Study the drawing (mm; zero at the part's minimum x, y, z) and answer. A direction names the side the tool comes from. Give positions to 0.01 mm unless a question says otherwise; leave off trailing zeros. Loops run counter-clockwise (first coordinate to the right, second up) from the corner with the lowest first, then second, coordinate; pieces in that order, holes last. Notation, with made-up numbers: M 50.25,77 L 109.25,77 A9 cw 109.25,90 Z; hole C 27.25,57.5 d6. An arc over 180 degrees is marked long. Return JSON: item names as keys, results as strings.
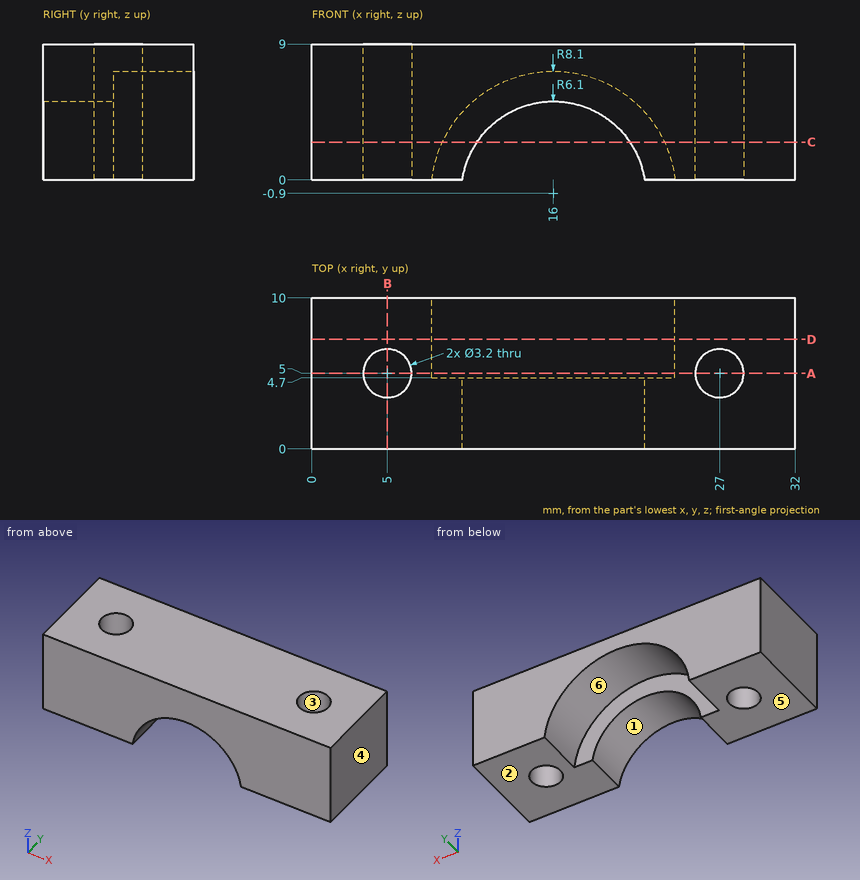
(1) Determine the mould class of the marked faces 1, 2, 3 and 4 for opening direction X: released by +X, released by -X, zero draft, split by the parting line, or undercut.
Values follow:
{"face 1": "undercut", "face 2": "zero draft", "face 3": "undercut", "face 4": "released by +X"}
(2) The part is cut by section D-D (y = 7.25). Determine the outline of the cut face in (x, z).
Values follow:
{"outline": "M 0,0 L 7.95,0 A8.1 cw 24.05,0 L 32,0 L 32,9 L 0,9 Z"}
(3) The part is cut by section C-C (z = 2.5). Determine the outline of the cut face in (x, y) (1 decimal).
Values follow:
{"outline": "M 0,0 L 10.9,0 L 10.9,4.7 L 8.6,4.7 L 8.6,10 L 0,10 Z; M 21.1,0 L 32,0 L 32,10 L 23.4,10 L 23.4,4.7 L 21.1,4.7 Z; hole C 5,5 d3.2; hole C 27,5 d3.2"}
(4) A tool of negligible diameter and unlimited length cuts with its end or side. For the marked faces 5 and 6, from which of +Z, -Z, +X, -X, +Y, -Y can it reach the whole face along a straight path? Write none if from no direction.
Values follow:
{"face 5": "-Z, +X, -X, +Y, -Y", "face 6": "-Z, +Y"}
(5) Given pin 1 (3 mm diameter, centred on x = 5, y = 5, fed in from +Z), flat-ended and moving along its own axis, determine where the tip first touches the part or whether it passes through.
Values follow:
{"pin 1": "through"}
(6) The part is cut by section B-B (x = 5). Determine the outline of the cut face in (y, z), and give its area (3 significant figures).
Values follow:
{"outline": "M 0,0 L 3.4,0 L 3.4,9 L 0,9 Z; M 6.6,0 L 10,0 L 10,9 L 6.6,9 Z", "area": "61.2 mm²"}
(7) The part is cut by section A-A (y = 5). Determine the outline of the cut face in (x, z), and give its area (3 significant figures).
Values follow:
{"outline": "M 0,0 L 3.4,0 L 3.4,9 L 0,9 Z; M 6.6,0 L 7.95,0 A8.1 cw 24.05,0 L 25.4,0 L 25.4,9 L 6.6,9 Z; M 28.6,0 L 32,0 L 32,9 L 28.6,9 Z", "area": "142 mm²"}
(8) Straight lines are drawn through the part: line 1 along Y through (x, z) = (5, 6.75); line 2 along X through (y, z) = (5.5, 7.75); line 3 along X through (y, z) = (8.25, 4.5). For each, find the intervals that lie inside material, in ascending order.
Values follow:
{"line 1": "0 to 3.4, 6.6 to 10", "line 2": "0 to 3.48, 6.52 to 25.48, 28.52 to 32", "line 3": "0 to 9.96, 22.04 to 32"}
